Drawing for the job (mm, zero at the part's lowest x, y, z). A direction names the side the tool comes from. Coordinates: 2 decimals unless noted, no trailing zeros. Order: outer loops, then holes, each group sorted by start corner. A loop starts at its lowest first (then second) coordinate and runs counter-clockwise, first axis right, second up.
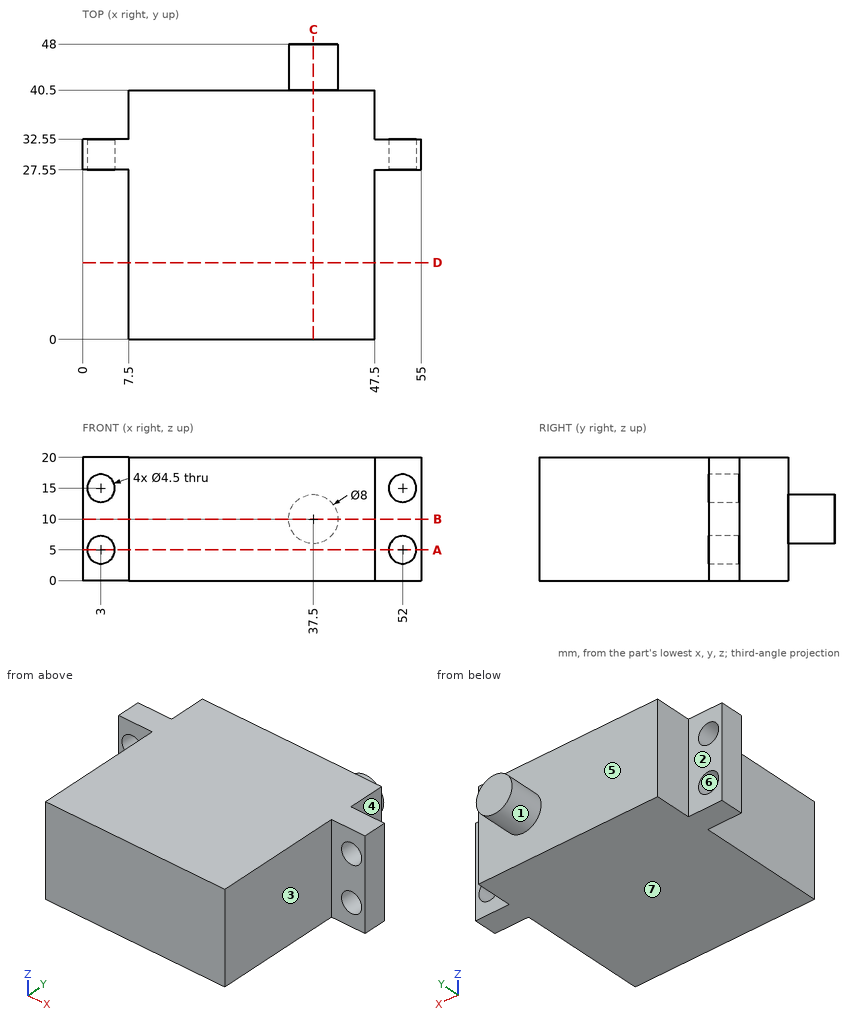
1) Slice it at C-C (x = 37.5). List the corners of the cut face in (y, z), plus the area to 3 significant figures.
2) Slice it at A-A (z = 5). List the corners of the cut face in (x, y), plus the area to 3 significant figures.
3) Slice it at D-D (y = 12.5). List the corners of the cut face in (x, z), plus the area to 3 significant figures.
4) Pin check, flat tips, straight feed: P1, Ø8, axis at x = 4, z = 12.5, coming from the +Y side; P2, Ø8.5, axis at y = 38.5, z = 6.5, coming from the +X side; P3, Ø2.5, axis at x = 3, z = 15, coming from the -Y side; P4, Ø5, axis at x = 52, z = 15, coming from the +Y side. Stop position of each tip, or through.
5) Slice it at B-B (z = 10). List the corners of the cut face in (x, y).
6) Two-plate mould, pull along Z, no slides. Class the marked faces 5, 6 and 7: released by +Z, released by -Z, zero draft, split by the parting line, or undercut.
7) Which spindle directions (+Z, -Z, +X, -X, +Y, -Y) get a long thin tool onto all of the face, cutting with end or side? Do the marked faces 1, 2, 3 and 4. Say none if no direction does.
8) Drill centre lines: probe 1 along X at (y, z) = (31.45, 5); probe 2 along Y at (x, z) = (19.5, 11.5); probe 3 along X at (y, z) = (31, 13.5). Where is each one in solid material? Low to high.
Worked out:
1. outline: (0, 0) - (40.5, 0) - (40.5, 6) - (48, 6) - (48, 14) - (40.5, 14) - (40.5, 20) - (0, 20) - close
1. area: 870 mm2
2. outline: (0, 27.55) - (0.75, 27.55) - (0.75, 32.55) - (0, 32.55) - close; (5.25, 27.55) - (7.5, 27.55) - (7.5, 0) - (47.5, 0) - (47.5, 27.55) - (49.75, 27.55) - (49.75, 32.55) - (47.5, 32.55) - (47.5, 40.5) - (7.5, 40.5) - (7.5, 32.55) - (5.25, 32.55) - close; (54.25, 27.55) - (55, 27.55) - (55, 32.55) - (54.25, 32.55) - close
2. area: 1,650 mm2
3. outline: (7.5, 0) - (47.5, 0) - (47.5, 20) - (7.5, 20) - close
3. area: 800 mm2
4. P1: stops at y = 40.5
4. P2: stops at x = 47.5
4. P3: passes through
4. P4: stops at y = 32.55
5. outline: (0, 27.55) - (7.5, 27.55) - (7.5, 0) - (47.5, 0) - (47.5, 27.55) - (55, 27.55) - (55, 32.55) - (47.5, 32.55) - (47.5, 40.5) - (41.5, 40.5) - (41.5, 48) - (33.5, 48) - (33.5, 40.5) - (7.5, 40.5) - (7.5, 32.55) - (0, 32.55) - close
6. face 5: zero draft
6. face 6: undercut
6. face 7: released by -Z
7. face 1: +Y
7. face 2: +Z, -Z, -X, +Y
7. face 3: +Z, -Z, +X, -Y
7. face 4: +Z, -Z, +X, +Y
8. probe 1: x = 0 to 0.75, 5.25 to 49.75, 54.25 to 55
8. probe 2: y = 0 to 40.5
8. probe 3: x = 0 to 1.32, 4.68 to 50.32, 53.68 to 55
